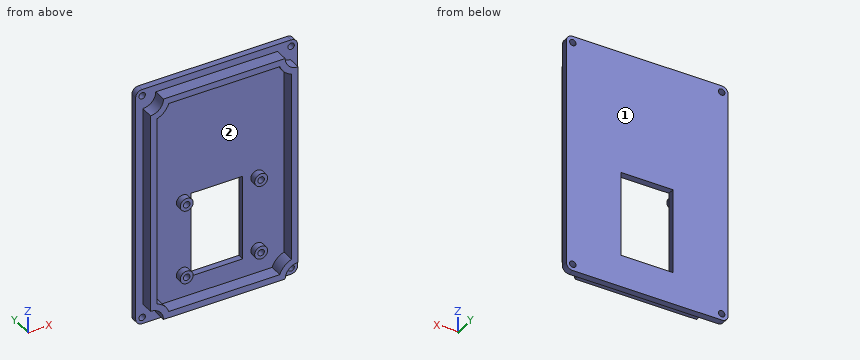
Autodesk Inventor part; units mm, degrees
ref_plane "YZ Plane" through (0, 0, 0) normal (1, 0, 0) x (0, 1, 0)
ref_plane "XZ Plane" through (0, 0, 0) normal (0, 1, 0) x (-1, 0, 0)
ref_plane "XY Plane" through (0, 0, 0) normal (0, 0, 1) x (1, 0, 0)
sketch "Sketch1" plane through (0, 0, 0) normal (0, 1, 0) x (-1, 0, 0)
  line L0 (25, 37.5) -> (-25, 37.5)
  line L1 (-25, 37.5) -> (-25, -37.5)
  line L2 (-25, -37.5) -> (25, -37.5)
  line L3 (25, -37.5) -> (25, 37.5)
  line L4 (-25, 37.5) -> (25, -37.5) construction
  circle A0 centre (23, -35.5) radius 1
  circle A1 centre (-23, -35.5) radius 1
  circle A2 centre (-23, 35.5) radius 1
  circle A3 centre (23, 35.5) radius 1
  point P0 (0, 0)
  point P1 (0, 0)
  dimension "d0" = 75
  dimension "d1" = 50
  dimension "d17" = 2
  dimension "d18" = 2
  dimension "d21" = 2
  dimension "d22" = 2
  dimension "d23" = 2
  dimension "d25" = 2
  dimension "d26" = 2
  dimension "d27" = 2
  dimension "d28" = 2
extrude "Extrusion1" add sketch "Sketch1" along normal blind 2
sketch "Sketch4" plane through (0, 0, 0) normal (0, -1, 0) x (1, 0, 0)
  line L0 (-18.8, 35.3) -> (18.8, 35.3)
  line L1 (22.8, 31.3) -> (22.8, -31.3)
  line L2 (18.8, -35.3) -> (-18.8, -35.3)
  line L3 (-22.8, -31.3) -> (-22.8, 31.3)
  line L4 (-22.8, 35.3) -> (22.8, -35.3) construction
  line L5 (-25, -37.5) -> (-25, 37.5)
  line L6 (-25, 37.5) -> (25, 37.5)
  arc A0 (-22.8, 31.3) -> (-18.8, 35.3) centre (-22.8, 35.3) ccw
  arc A1 (18.8, 35.3) -> (22.8, 31.3) centre (22.8, 35.3) ccw
  arc A2 (-18.8, -35.3) -> (-22.8, -31.3) centre (-22.8, -35.3) ccw
  arc A3 (22.8, -31.3) -> (18.8, -35.3) centre (22.8, -35.3) ccw
  line L7 (17.1431, 33.3) -> (-17.1431, 33.3)
  arc A4 (-20.8, 29.6431) -> (-17.1431, 33.3) centre (-22.8, 35.3) ccw
  line L8 (-20.8, 29.6431) -> (-20.8, -29.6431)
  arc A5 (-17.1431, -33.3) -> (-20.8, -29.6431) centre (-22.8, -35.3) ccw
  line L9 (-17.1431, -33.3) -> (17.1431, -33.3)
  arc A6 (20.8, -29.6431) -> (17.1431, -33.3) centre (22.8, -35.3) ccw
  line L10 (20.8, -29.6431) -> (20.8, 29.6431)
  arc A7 (17.1431, 33.3) -> (20.8, 29.6431) centre (22.8, 35.3) ccw
  point P0 (0, 0)
  point P1 (0, 0)
  dimension "d29" = 2.2
  dimension "d30" = 2.2
  dimension "d32" = 4
  dimension "d35" = 2
extrude "Extrusion4" add sketch "Sketch4" along normal blind 4
sketch "Sketch5" plane through (0, 0, 0) normal (0, -1, 0) x (1, 0, 0)
  line L0 (-10.4342, -25.835) -> (12.5658, -25.835) construction
  line L1 (12.5658, -25.835) -> (12.5658, -2.585) construction
  line L2 (12.5658, -2.585) -> (-10.4342, -2.585) construction
  line L3 (-10.4342, -2.585) -> (-10.4342, -25.835) construction
  line L4 (-10.4342, -2.585) -> (12.5658, -25.835) construction
  circle A0 centre (-10.4342, -2.585) radius 1
  circle A1 centre (-10.4342, -25.835) radius 1
  circle A2 centre (12.5658, -25.835) radius 1
  circle A3 centre (12.5658, -2.585) radius 1
  circle A4 centre (-10.4342, -25.835) radius 2
  circle A5 centre (-10.4342, -2.585) radius 2
  circle A6 centre (12.5658, -2.585) radius 2
  circle A7 centre (12.5658, -25.835) radius 2
  line L5 (-10.4342, -14.21) -> (12.5658, -14.21) construction
  point P0 (0, 0)
  dimension "d36" = 23.25
  dimension "d37" = 23
  dimension "d38" = 2
  dimension "d39" = 4
extrude "Extrusion5" add sketch "Sketch5" along normal blind 2
sketch "Sketch6" plane through (0, 0, 0) normal (0, -1, 0) x (1, 0, 0)
  line L0 (-7.9342, -27.46) -> (8.0658, -27.46)
  line L1 (8.0658, -27.46) -> (8.0658, -0.96)
  line L2 (8.0658, -0.96) -> (-7.9342, -0.96)
  line L3 (-7.9342, -0.96) -> (-7.9342, -27.46)
  circle A0 centre (-10.4342, -25.835) radius 1
  line L4 (-10.58, -24.8457) -> (-10.58, -3.5743) construction
  circle A1 centre (-10.4342, -2.585) radius 1
  line L5 (-10.58, -14.21) -> (-1.6995, -14.21) construction
  point P0 (0, 0)
  dimension "d42" = 16
  dimension "d43" = 26.5
  dimension "d45" = 1.5
extrude "Extrusion6" cut sketch "Sketch6" against normal blind 10 contours L3 L2 L1 L0
fillet "Fillet2" radius 2 4 edges at (-25, 1, 37.5) (-25, 1, -37.5) (25, 1, -37.5) (25, 1, 37.5)
equation "\"d18\" = d17"
equation "\"d22\" = d17"
equation "\"d23\" = d17"
equation "\"d25\" = d17"
equation "\"d26\" = d17"
equation "\"d27\" = d17"
equation "\"d28\" = d17"
equation "\"d30\" = d29"
properties part number "Enclosure Lid"
Design review of the part built by this model. Coordinates are the model's own, in mm. Face numbers are marked on the shaded views. Round coordinates to 2 decimals unless told otherwise and drop trailing zeros. Write each loop counter-clockwise with the first axis right and the second up, starting at its lowest first coordinate (ties: lowest second). Pieces come first, ordered by that corner, then holes.
Item 1: Clearance check with flat-ended pins moving along their axes: pin 1 Ø1 at (x, y) = (-16, -3) entering from +Z; pin 2 Ø3 at (x, z) = (-10, -2) entering from -Y; pin 3 Ø0.6 at (x, z) = (12.5, -2.5) entering from -Y; pin 4 Ø1.2 at (x, z) = (23, -35.5) entering from +Y. State where each tip first meets the part, or that it passes through.
Item 2: We need section D-D on z = -32.5. Write out the cut boundary in (x, y), and give its area (3 significant figures).
Item 3: We need section A-A on z = -19.5. Write out the cut boundary in (x, y), and give its area (3 significant figures).
Item 4: For probe 1 along Z at (x, y) = (23, 1.45); probe 2 along Z at (x, y) = (0.5, -1.6); probe 3 along X at (y, z) = (-2.55, -28), list the stretches that pass through material, from the lowest coordinate up.
Item 5: The part is to be moulded in two halves that separate along X. For the marked faces 1 and 2, say which applies: +X half, -X half, draft (parallel to the pull), parting line (faces both ways), or undercut.
Item 6: We need section C-C on z = 5.5. Write out the cut boundary in (x, y), and give its area (3 significant figures).
Item 7: We need section B-B on y = -1.15. State how many separate pieces and enclosed holes the cut face has, and give its area (3 significant figures).
Returned:
1. pin 1: stops at z = 35.3
1. pin 2: stops at y = -2
1. pin 3: stops at y = 0
1. pin 4: passes through
2. outline: (-25, 0) - (-19.94, 0) - (-19.94, -4) - (-17.49, -4) - (-17.49, 0) - (17.49, 0) - (17.49, -4) - (19.94, -4) - (19.94, 0) - (25, 0) - (25, 2) - (-25, 2) - close
2. area: 120 mm2
3. outline: (-25, 0) - (-22.8, 0) - (-22.8, -4) - (-20.8, -4) - (-20.8, 0) - (-7.93, 0) - (-7.93, 2) - (-25, 2) - close; (8.07, 0) - (20.8, 0) - (20.8, -4) - (22.8, -4) - (22.8, 0) - (25, 0) - (25, 2) - (8.07, 2) - close
3. area: 84.0 mm2
4. probe 1: z = -37.5 to -36.5, -34.5 to 34.5, 36.5 to 37.5
4. probe 2: z = -35.3 to -33.3, 33.3 to 35.3
4. probe 3: x = -22.8 to -20.8, 20.8 to 22.8
5. face 1: draft
5. face 2: undercut
6. outline: (-25, 0) - (-22.8, 0) - (-22.8, -4) - (-20.8, -4) - (-20.8, 0) - (20.8, 0) - (20.8, -4) - (22.8, -4) - (22.8, 0) - (25, 0) - (25, 2) - (-25, 2) - close
6. area: 116 mm2
7. separate pieces: 5
7. enclosed holes: 5
7. area: 471 mm2
